Could you check a few things on this model? Use its own coordinates, in mm. Face numbers are marked on the shaded views. A direction names the side the tool comes from. Give positions to 0.01 mm unless a question says otherwise; leave off trailing zeros. Order: outer loops, then holes, each group sorted by start corner. A loop starts at its lowest first (then second) coordinate and runs counter-clockwise, first axis right, second up. Notation, with made-up numbers: M 86.25,21.25 L 138.25,21.25 A36 ccw 138.25,58.25 Z; hole C 23,-29.75 d8. An arc over 180 degrees is marked long. Return JSON: item names as keys, results as strings. Group by question number.
```python
from build123d import *

# Parameters (mm, degrees)
F1_DEPTH = 25
F2_R     = 5
F3_R     = 9.898276
F4_R     = 1
F5_R     = 6.5
F6_DEPTH = 3
F8_DEPTH = 1


with BuildPart() as f1:
    # F0 (on Top) → F1 (new body)
    with BuildSketch(Plane.XY):
        with BuildLine():
            ThreePointArc((30.5, 0), (15.25, -15.25), (0, 0))
            Line((0, 0), (0, 20))
            ThreePointArc((0, 20), (4.466622, 30.783378), (15.25, 35.25))
            Line((15.25, 35.25), (3.50266, 35.25))
            ThreePointArc((3.50266, 35.25), (-2.022794, 28.497829), (-4, 20))
            Line((-4, 20), (-4, 0))
            Line((-4, 0), (-34, 0))
            Line((-34, 0), (-40.494669, 6.624704))
            Line((-40.494669, 6.624704), (-43.350991, 3.824449))
            Line((-43.350991, 3.824449), (-35.680126, -4))
            Line((-35.680126, -4), (-3.57983, -4))
            ThreePointArc((-3.57983, -4), (17.261004, -19.144669), (34.5, 0))
            Line((34.5, 0), (30.5, 0))
        make_face()
    extrude(amount=F1_DEPTH)

    # F2
    f2_edges = [f1.edges().sort_by_distance(p)[0] for p in [
        (-35.680126, -4, 12.5),
        (-34, 0, 12.5),
    ]]
    fillet(f2_edges, radius=F2_R)

    # F3
    f3_edges = [f1.edges().sort_by_distance(p)[0] for p in [
        (-3.57983, -4, 12.5),
        (-4, 0, 12.5),
    ]]
    fillet(f3_edges, radius=F3_R)

    # F4
    f4_edges = [f1.edges().sort_by_distance(p)[0] for p in [
        (34.5, 0, 12.5),
        (32.5, 0, 25),
        (32.5, 0, 0),
        (3.50266, 35.25, 12.5),
    ]]
    fillet(f4_edges, radius=F4_R)

    # F5 (on face) → F6 (cut)
    with BuildSketch(Plane.YZ):
        with Locations((13.5, 12.5)):
            Circle(F5_R)
    extrude(amount=-F6_DEPTH, mode=Mode.SUBTRACT)

    # F7 (on face) → F8 (join)
    with BuildSketch(Plane(origin=(0, 0, 0), x_dir=(1, 0, 0), z_dir=(0, 0, -1))):
        Polygon((-42.2277, 8.48738), (-39.850672, -0.254048), (-33.792032, -6.193764), (-28.426796, -4.05625), (-30.911811, 8.48738), align=None)
    extrude(amount=-F8_DEPTH)


solid = f1.part
```
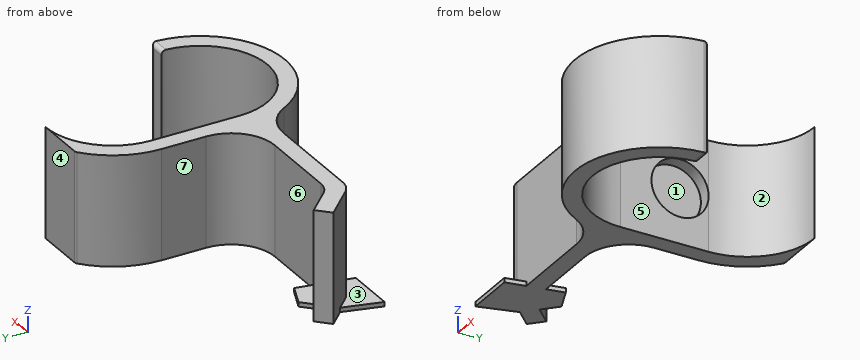
1. I need wall thicknesses on L1, parallel to Z at x = -2.35, y = 13.5; L2, parallel to X at y = 9.5, z = 17.5; L3, parallel to X at y = 18, z = 20.5. Which ranges of each line are inside material? Lowest first, please. Write a range as from..to.
2. Imagine slicing it at B-B, the plane z = 3.5. Please give me the cut outline in (x, y).
3. Imagine slicing it at C-C, the plane x = 10.5. Please give me the cut outline in (y, z), plus the area to 3 significant figures.
4. Imagine slicing it at D-D, the plane y = 19. Please give me the cut outline in (x, z).
5. If we mould it in two halves opening along X, with no side actions, what happens to the marked faces 4, 5, 6 and 7? For each: pulls with the +X half, pulls with the -X half, needs draft (parallel to the pull), parting line crosses it, or undercut.
6. For pin 1 (9 mm diameter, centred on x = -25.5, z = 6.5, fed in from +Y); pin 2 (2 mm diameter, centred on x = -20.5, z = 7, fed in from -Y); pin 3 (6 mm diameter, centred on y = 10, z = 7.5, fed in from +X), each with a flat end and sliding along its axis, tell me the tip position at first contact or that it passes through.
7. Imagine slicing it at A-A, the plane y = 13.5. Please give me the cut outline in (x, z), plus the area to 3 significant figures.
8. Which directions (+Z, -Z, +X, -X, +Y, -Y) give clear straight access to the entire face, cutting with the end or side of a thin tool? Please do the marked faces 1, 2 and 3.
Values:
{
 "1": {"L1": "z = 0..6, 19..25", "L2": "x = -4.01..-3", "L3": "x = -4..0"},
 "2": {"outline": "M -43.35,3.82 L -37.15,-2.5 A5 ccw -33.58,-4 L -10.37,-4 A9.9 cw -1.67,-9.18 A19.25 ccw 34.47,-1.05 A1 ccw 33.47,0 L 30.5,0 A15.25 cw 0,0 L 0,20 A15.25 cw 15.25,35.25 L 3.85,35.25 A1 ccw 3.22,35.03 A19.25 ccw -4,20 L -4,9.9 A9.9 cw -13.9,0 L -31.9,0 A5 cw -35.47,1.5 L -40.49,6.62 Z"},
 "3": {"outline": "M -18.65,0 L -14.49,0 L -14.49,25 L -18.65,25 Z; M 34.49,0 L 35.25,0 L 35.25,25 L 34.49,25 Z", "area": "123 mm²"},
 "4": {"outline": "M -4,0 L 0,0 L 0,9.04 L -3,9.04 L -3,15.96 L 0,15.96 L 0,25 L -4,25 Z"},
 "5": {"face 4": "needs draft", "face 5": "pulls with the +X half", "face 6": "undercut", "face 7": "pulls with the -X half"},
 "6": {"pin 1": "stops at y = 0", "pin 2": "stops at y = -4", "pin 3": "stops at x = 0"},
 "7": {"outline": "M -4,0 L 0,0 L 0,6 L -3,6 L -3,19 L 0,19 L 0,25 L -4,25 Z", "area": "61.0 mm²"},
 "8": {"face 1": "+X", "face 2": "+Z, -Z, +X", "face 3": "+Z, -X, -Y"}
}
